Can you work these out from the model? Positions are in its coordinate system, mm. A direction names the side the tool comes from. Give positions to 0.01 mm unless a question says otherwise; leave off trailing zeros. Order: outer loops, then holes, each group sorted by start corner. A loop starts at its lowest first (then second) coordinate and runs counter-clockwise, first axis right, second up. Notation, with made-up numbers: (70.25, 12.25) - (103.25, 12.25) arc R38 ccw to (103.25, 51.25) - close; hole circle Ø4 at (59, 42). An arc over 180 degrees is marked (long way). One line per question, with ' | ' between items.
```python
from build123d import *

# Parameters (mm, degrees)
F0_W     = 400
F0_H     = 200
F1_DEPTH = 11
F2_R     = 5
F2_R_2   = 80
F3_DEPTH = 7
F2_W     = 200
F2_H     = 200
F2_R_3   = 77
F4_DEPTH = 5


with BuildPart() as f1:
    # F0 (on Top) → F1 (new body)
    with BuildSketch(Plane.XY):
        with Locations((164.849856, 81.428634)):
            Rectangle(F0_W, F0_H)
    extrude(amount=F1_DEPTH)

    # F2 (on face) → F3 (cut)
    with BuildSketch(Plane.XY.offset(11)):
        with Locations((-25.150144, -8.558058)):
            Circle(F2_R)
        with Locations((64.849856, 81.428634)):
            Circle(F2_R_2)
        with Locations((-25.209671, 171.52901)):
            Circle(F2_R)
    extrude(amount=-F3_DEPTH, mode=Mode.SUBTRACT)

    # F2 (on face) → F4 (cut)
    with BuildSketch(Plane.XY.offset(11)):
        with Locations((264.849856, 81.428634)):
            Rectangle(F2_W, F2_H)
        with Locations((354.849856, -8.558058)):
            Circle(F2_R, mode=Mode.SUBTRACT)
        with Locations((264.849856, 81.428634)):
            Circle(F2_R_3, mode=Mode.SUBTRACT)
        with Locations((354.909382, 171.52901)):
            Circle(F2_R, mode=Mode.SUBTRACT)
    extrude(amount=-F4_DEPTH, mode=Mode.SUBTRACT)


solid = f1.part
```
(1) Imagine slicing it at A-A (z = 8.25). List the corners of the cut face in (x, y) for me.
Answer below:
outline: (-35.15, -18.57) - (164.85, -18.57) - (164.85, 181.43) - (-35.15, 181.43) - close; circle Ø154 at (264.85, 81.43); circle Ø10 at (354.85, -8.56); circle Ø10 at (354.91, 171.53); hole circle Ø10 at (-25.21, 171.53); hole circle Ø10 at (-25.15, -8.56); hole circle Ø160 at (64.85, 81.43)
(2) Imagine slicing it at B-B (y = 100.5). List the corners of the cut face in (x, z) for me.
Answer below:
outline: (-35.15, 0) - (364.85, 0) - (364.85, 6) - (339.45, 6) - (339.45, 11) - (190.25, 11) - (190.25, 6) - (164.85, 6) - (164.85, 11) - (142.54, 11) - (142.54, 4) - (-12.84, 4) - (-12.84, 11) - (-35.15, 11) - close
(3) Imagine slicing it at D-D (y = 56.5). List the corners of the cut face in (x, z) for me, and give its area (3 significant figures).
Answer below:
outline: (-35.15, 0) - (364.85, 0) - (364.85, 6) - (337.7, 6) - (337.7, 11) - (192, 11) - (192, 6) - (164.85, 6) - (164.85, 11) - (140.87, 11) - (140.87, 4) - (-11.17, 4) - (-11.17, 11) - (-35.15, 11) - close | area: 3,060 mm^2
(4) Will this pin go through, and if not, where does the flat tip stop? pin 1 (6 mm diameter, centred on x = -25.21, y = 171.53, fed in from +Z).
Answer below:
pin 1: z = 4
(5) If we mould it in two halves opening along X, with no side actions, what happens to faces 3 (the face through (359.47, -10.47, 8.54)), 4 (the face through (-35.15, 80, 5)), 5 (the face through (108, 149, 11)), 6 (the face through (-25, 172, 4))? For each: released by +X, released by -X, zero draft, split by the parting line, or undercut.
Answer below:
face 3: undercut | face 4: released by -X | face 5: zero draft | face 6: undercut
(6) On a 3-axis mill with a long thin cutter (end or side, diameter ignored), from which of +Z, -Z, +X, -X, +Y, -Y can I reach the whole of each face in a straight line? I mean faces 1 (the face through (-26.23, -13.44, 7.55)), 2 (the face through (118, -18.571, 4)). Say none if no direction works.
Answer below:
face 1: +Z | face 2: +Z, -Z, +X, -X, -Y
(7) Imagine slicing it at C-C (x = 192.5). List the corners of the cut face in (y, z) for me, and give its area (3 significant figures).
Answer below:
outline: (-18.57, 0) - (181.43, 0) - (181.43, 6) - (107.78, 6) - (107.78, 11) - (55.08, 11) - (55.08, 6) - (-18.57, 6) - close | area: 1,460 mm^2
(8) If I drill on line 1 (X direction, y = 81.5, z = 6.25); line 2 (X direction, y = 171.5, z = 7.75); line 3 (Z direction, x = 340.5, y = 137), over which ranges is the centre line in solid material (lowest first)?
Answer below:
line 1: -35.15 to -15.15, 144.85 to 164.85, 187.85 to 341.85 | line 2: -35.15 to -30.21, -20.21 to 164.85, 349.91 to 359.91 | line 3: 0 to 6
